Check sheet for the modelled part. Datum: model origin and axes. Units: mm. A direction names the side the tool comes from. Round coordinates to 2 decimals unless told otherwise and drop trailing zeros. Order: outer loops, then holes, each group sorted by start corner. A loop starts at its lowest first (then second) coordinate and runs counter-clockwise, first axis right, second up.
Autodesk Inventor part; units mm, degrees
ref_plane "YZ Plane" through (0, 0, 0) normal (1, 0, 0) x (0, 1, 0)
ref_plane "XZ Plane" through (0, 0, 0) normal (0, 1, 0) x (-1, 0, 0)
ref_plane "XY Plane" through (0, 0, 0) normal (0, 0, 1) x (1, 0, 0)
sketch "Sketch1" plane through (0, 0, 0) normal (0, 0, 1) x (1, 0, 0)
  line L0 (17.5, -17.5) -> (0, -17.5)
  line L1 (-17.5, -17.5) -> (-17.5, 17.5)
  line L2 (-17.5, 17.5) -> (-7.5, 17.5) construction
  line L3 (17.5, 17.5) -> (17.5, 10)
  line L4 (17.5, -17.5) -> (-17.5, 17.5) construction
  line L5 (-17.5, -17.5) -> (17.5, 17.5) construction
  line L6 (-17.5, -17.5) -> (-21.5, -17.5)
  line L7 (-21.5, -17.5) -> (-21.5, -7.5)
  line L8 (-21.5, -7.5) -> (-17.5, -7.5)
  line L9 (-17.5, -7.5) -> (-17.5, -17.5) construction
  line L10 (-17.5, 0) -> (-21.5, 0)
  line L11 (-21.5, 0) -> (-21.5, 10)
  line L12 (-21.5, 10) -> (-17.5, 10)
  line L13 (-17.5, 10) -> (-17.5, 0) construction
  line L14 (-17.5, 17.5) -> (-7.5, 17.5) construction
  line L15 (-7.5, 17.5) -> (-7.5, 21.5)
  line L16 (-7.5, 21.5) -> (-17.5, 21.5)
  line L17 (-17.5, 21.5) -> (-17.5, 17.5)
  line L18 (0, 17.5) -> (10, 17.5) construction
  line L19 (10, 17.5) -> (10, 21.5)
  line L20 (10, 21.5) -> (0, 21.5)
  line L21 (0, 21.5) -> (0, 17.5)
  line L22 (-17.5, 0) -> (17.5, 0) construction
  line L23 (0, -17.5) -> (0, 17.5) construction
  line L24 (-17.5, -17.5) -> (-7.5, -17.5)
  line L25 (-7.5, -17.5) -> (-7.5, -21.5)
  line L26 (-7.5, -21.5) -> (-17.5, -21.5)
  line L27 (-17.5, -21.5) -> (-17.5, -17.5)
  line L28 (0, -17.5) -> (10, -17.5) construction
  line L29 (10, -17.5) -> (10, -21.5)
  line L30 (10, -21.5) -> (0, -21.5)
  line L31 (0, -21.5) -> (0, -17.5)
  line L32 (17.5, -17.5) -> (21.5, -17.5)
  line L33 (21.5, -17.5) -> (21.5, -7.5)
  line L34 (21.5, -7.5) -> (17.5, -7.5)
  line L35 (17.5, -7.5) -> (17.5, -17.5) construction
  line L36 (17.5, 0) -> (21.5, 0)
  line L37 (21.5, 0) -> (21.5, 10)
  line L38 (21.5, 10) -> (17.5, 10)
  line L39 (17.5, 10) -> (17.5, 0) construction
  line L40 (-7.5, 17.5) -> (0, 17.5)
  line L41 (0, 17.5) -> (10, 17.5)
  line L42 (17.5, 10) -> (17.5, 0) construction
  line L43 (17.5, 0) -> (17.5, -7.5)
  line L44 (17.5, -7.5) -> (17.5, -17.5) construction
  line L45 (0, -17.5) -> (-17.5, -17.5)
  line L46 (10, 17.5) -> (17.5, 17.5)
  point P0 (0, 0)
  point P1 (0, 19.5)
  point P2 (-7.5, 19.5)
  point P3 (0, -19.5)
  point P4 (-7.5, -19.5)
  point P5 (-17.5, -7.5)
  point P6 (10, -17.5)
  dimension "d5" = 10
  dimension "d6" = 10
  dimension "d7" = 7.5
  dimension "d8" = 4
  dimension "d9" = 10
  dimension "d10" = 4
  dimension "d11" = 10
  dimension "d12" = 4
  dimension "d13" = 7.5
  dimension "d16" = 35
  dimension "d17" = 35
extrude "Extrusion1" add sketch "Sketch1" along normal blind 4
sketch "Sketch2" plane through (0, 0, 0) normal (0, 0, -1) x (-1, 0, 0)
  line L0 (-3.5, 17.5) -> (-6.5, 17.5) construction
  line L1 (-3.5, 21.5) -> (-3.5, 17.5) construction
  line L2 (-6.5, 21.5) -> (-3.5, 21.5) construction
  line L3 (-6.5, 21.5) -> (-6.5, 17.5) construction
  line L4 (-3.5, -21.5) -> (-6.5, -21.5) construction
  line L5 (-3.5, -17.5) -> (-3.5, -21.5) construction
  line L6 (-6.5, -17.5) -> (-3.5, -17.5) construction
  line L7 (-6.5, -17.5) -> (-6.5, -21.5) construction
  line L8 (-6.5, 21.5) -> (-3.5, 17.5) construction
  line L9 (-6.5, -21.5) -> (-3.5, -17.5) construction
  circle A0 centre (-5, 19.5) radius 1.5
  circle A1 centre (-5, -19.5) radius 1.5
  point P0 (0, 0)
  dimension "d18" = 3
extrude "Extrusion2" cut sketch "Sketch2" against normal up to next
properties part number "FloorButtonHolder_Back_V1" material "MDF Medium Density Fiberboard"
Item 1: Release check for a two-part mould opening along Y. For faces 4 (the flat face through (-4, 17.5, 2)), 5 (the flat face through (19, 0, 2)), 6 (the flat face through (-20, -7.5, 2)), 7 (the flat face through (5, -21.5, 2)) record: released by +Y, released by -Y, zero draft, split by the parting line, or undercut.
Answer:
face 4: released by +Y
face 5: undercut
face 6: undercut
face 7: released by -Y
Item 2: Go/stop test with flat-tipped pins: P1, Ø2, axis at x = 12, z = 1.5, coming from the +Y side; P2, Ø2, axis at y = 20, z = 2.5, coming from the +X side; P3, Ø1.2, axis at x = 15, z = 2, coming from the -Y side. Record where each tip stops, or that it passes through.
Answer:
P1: stops at y = 17.5
P2: stops at x = 10
P3: stops at y = -17.5
Item 3: Sectioned sample at B-B (x = 5). Record the cut outline in (y, z), and give its area (3 significant figures).
Answer:
outline: (-21.5, 0) - (-21, 0) - (-21, 4) - (-21.5, 4) - close; (-18, 0) - (18, 0) - (18, 4) - (-18, 4) - close; (21, 0) - (21.5, 0) - (21.5, 4) - (21, 4) - close
area: 148 mm2
Item 4: Sectioned sample at A-A (z = 3). State how many separate pieces and enclosed holes the cut face has, and give its area (3 significant figures).
Answer:
separate pieces: 1
enclosed holes: 2
area: 1,530 mm2
Item 5: Sectioned sample at D-D (x = 17). Record the cut outline in (y, z), and give its area (3 significant figures).
Answer:
outline: (-17.5, 0) - (17.5, 0) - (17.5, 4) - (-17.5, 4) - close
area: 140 mm2
Item 6: Scan lines: line 1 along Y through (x, z) = (5, 1.8); line 2 along Y through (x, z) = (5.5, 1.15); line 3 along Y through (x, z) = (20.5, 1.35). Record each from-to range of solid material in increasing order.
Answer:
line 1: y = -21.5 to -21, -18 to 18, 21 to 21.5
line 2: y = -21.5 to -20.91, -18.09 to 18.09, 20.91 to 21.5
line 3: y = -17.5 to -7.5, 0 to 10
Item 7: Access from +Z, -Z, +X, -X, +Y, -Y to the whole of each face (thin tool, end or side, straight path). Record for faces 1 (the flat face through (20, -7.5, 2)), 2 (the flat face through (-17.5, 16, 2)), 3 (the flat face through (-4, -17.5, 2)).
Answer:
face 1: +Z, -Z, +X
face 2: +Z, -Z, -X, +Y
face 3: +Z, -Z, -Y
Item 8: Sectioned sample at C-C (y = 19.5). Record the cut outline in (x, z).
Answer:
outline: (-17.5, 0) - (-7.5, 0) - (-7.5, 4) - (-17.5, 4) - close; (0, 0) - (3.5, 0) - (3.5, 4) - (0, 4) - close; (6.5, 0) - (10, 0) - (10, 4) - (6.5, 4) - close
